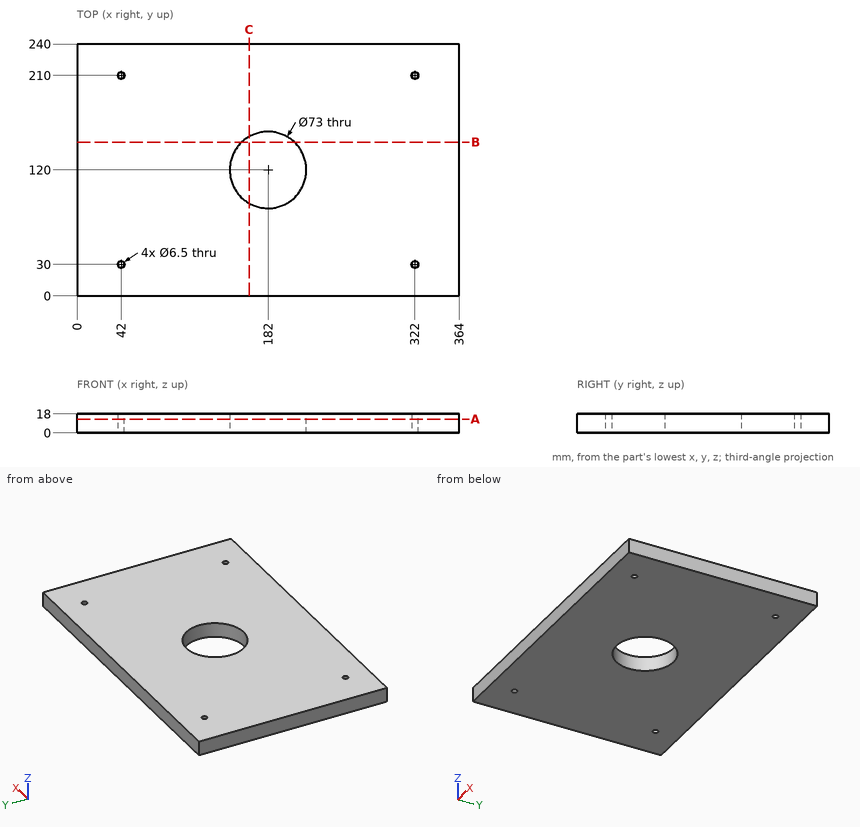
Verification items for this drawing (mm, ordinates from the low corner). Give positions to 0.01 mm unless a question says otherwise; leave off trailing zeros. Write each loop counter-clockwise with the first axis right and the second up, starting at its lowest first coordinate (ties: lowest second). Pieces come first, ordered by that corner, then holes. Notation, with made-up numbers: M 61.25,56 L 96.25,56 A27 cw 96.25,81 Z; hole C -35.5,-32.5 d6. An arc over 180 degrees is marked long. Use one line per item in the form item = value.
(1) Depth check by flat-ended pin: P1, Ø7.5, axis at x = 322, y = 30, coming from the +Z side; P2, Ø4, axis at x = 322, y = 210, coming from the +Z side. Enter the tip coordinate at first touch or a pass-through.
Answer block:
P1 = 18
P2 = through
(2) Material ranges on line 1 along X through (y, z) = (30, 11.25); line 2 along Y through (x, z) = (322, 10.75); line 3 along Y through (x, z) = (184, 4), recorded low to high.
Answer block:
line_1 = 0 to 38.75, 45.25 to 318.75, 325.25 to 364
line_2 = 0 to 26.75, 33.25 to 206.75, 213.25 to 240
line_3 = 0 to 83.55, 156.45 to 240
(3) Section check A-A on z = 13. Record the boundary of the cut face in (x, y).
Answer block:
outline = M 0,0 L 364,0 L 364,240 L 0,240 Z; hole C 42,30 d6.5; hole C 42,210 d6.5; hole C 182,120 d73; hole C 322,30 d6.5; hole C 322,210 d6.5
(4) Section check C-C on x = 164. Record the boundary of the cut face in (y, z).
Answer block:
outline = M 0,0 L 88.25,0 L 88.25,18 L 0,18 Z; M 151.75,0 L 240,0 L 240,18 L 151.75,18 Z
(5) Section check B-B on y = 146.5. Record the boundary of the cut face in (x, z), plus the area to 3 significant figures.
Answer block:
outline = M 0,0 L 156.9,0 L 156.9,18 L 0,18 Z; M 207.1,0 L 364,0 L 364,18 L 207.1,18 Z
area = 5,650 mm2
